from build123d import *

# Parameters (mm, degrees)
SCHIZZO1_R                   = 1.75
SCHIZZO1_R_2                 = 12.1
ESTRUSIONE_ESTRUSIONE1_DEPTH = 1
ESTRUSIONE_ESTRUSIONE2_START = -1.8
SCHIZZO2_R                   = 12.1
SCHIZZO2_R_2                 = 9
ESTRUSIONE_ESTRUSIONE2_DEPTH = 1.8


with BuildPart() as part:
    # Schizzo1 → Estrusione-Estrusione1 (new body)
    with BuildSketch(Plane.XY):
        with BuildLine():
            Line((-10.957517396, -18.677002221), (10.886206072, -18.677002221))
            ThreePointArc((10.886206072, -18.677002221), (14.572915114, -17.149917336), (16.1, -13.463208293))
            Line((16.1, -13.463208293), (16.1, 4.907883736))
            ThreePointArc((16.1, 4.907883736), (13.651991863, 12.73622021), (6.171311325, 16.1))
            Line((6.171311325, 16.1), (-6.171311325, 16.1))
            ThreePointArc((-6.171311325, 16.1), (-13.242379137, 13.171067812), (-16.171311325, 6.1))
            Line((-16.171311325, 6.1), (-16.171311325, -13.463208293))
            ThreePointArc((-16.171311325, -13.463208293), (-14.644226439, -17.149917336), (-10.957517396, -18.677002221))
        make_face()
        with Locations((0, -15.38859776)):
            Circle(SCHIZZO1_R, mode=Mode.SUBTRACT)
        with Locations((10.944459062, 10.817992606)):
            Circle(SCHIZZO1_R, mode=Mode.SUBTRACT)
        with Locations((-10.910719744, 10.851964601)):
            Circle(SCHIZZO1_R, mode=Mode.SUBTRACT)
        Circle(SCHIZZO1_R_2, mode=Mode.SUBTRACT)
    extrude(amount=ESTRUSIONE_ESTRUSIONE1_DEPTH)

    # Schizzo2 → Estrusione-Estrusione2 (add)
    with BuildSketch(Plane.XY.offset(1).offset(ESTRUSIONE_ESTRUSIONE2_START)):
        Circle(SCHIZZO2_R)
        Circle(SCHIZZO2_R_2, mode=Mode.SUBTRACT)
    extrude(amount=ESTRUSIONE_ESTRUSIONE2_DEPTH)


solid = part.part
Work out the finished part from the listing and answer in its coordinate system (mm). A direction names the side the tool comes from. Give positions to 0.01 mm unless a question says otherwise; leave off trailing zeros. Order: outer loops, then holes, each group sorted by start corner. A loop starts at its lowest first (then second) coordinate and runs counter-clockwise, first axis right, second up. Notation, with made-up numbers: (80.25, 27) -> (99.25, 27) arc R24 ccw to (99.25, 50) -> close; hole circle Ø4 at (-17.75, -39). An arc over 180 degrees is marked (long way). Answer as a JSON object with one key per item and string values. Group by question number.
1. Section D-D on x = -8 is taken. Determine the outline of the cut face in (y, z).
2. Section C-C on z = 0.35 is taken. Determine the outline of the cut face in (x, y).
3. A tool of negligible diameter and unlimited length cuts with its end or side. For faces 1 (the flat face through (0.1, 16.1, 0.5)), 2 (the flat face through (0, -13, 0)), 3 (the flat face through (16.1, -4.4, 0.5)), from which of +Z, -Z, +X, -X, +Y, -Y can it reach the whole face along a straight path? Write none if from no direction.
4. Consider line 1 along Y through (x, z) = (0, 0.5); line 2 along Z through (x, y) = (-9, -16); line 3 along X through (y, z) = (11, 0.65). Determine where each line is inside the solid, lowest interval first. Write a range as [from, to].
5. Section A-A on x = 0 is taken. Determine the outline of the cut face in (y, z).
6. Section B-B on y = 0 is taken. Determine the outline of the cut face in (x, z), plus the area to 3 significant figures.
7. Flat-ended cylindrical pins translate along their axes: pin 1 Ø3 at (x, y) = (-10.91, 10.85) entering from -Z; pin 2 Ø4 at (x, y) = (0, -15.39) entering from -Z; pin 3 Ø0.8 at (y, z) = (-8, 0.5) entering from +X. Find the tip coordinate at first contact, or state that the pin passes through.
8. The mould has two halves that part along X. Classify faces 4 (the cylindrical face through (-14.685, -17.109, 0.493)), 5 (the cylindrical face through (-0.228, -13.653, 0.493)), 6 (the flat face through (3, -9, 1)): released by +X, released by -X, zero draft, split by the parting line, or undercut.
Result sheet:
{
 "1": {"outline": "(-18.68, 0) -> (-9.08, 0) -> (-9.08, -0.8) -> (-4.12, -0.8) -> (-4.12, 1) -> (-18.68, 1) -> close; (4.12, -0.8) -> (9.08, -0.8) -> (9.08, 0) -> (15.93, 0) -> (15.93, 1) -> (4.12, 1) -> close"},
 "2": {"outline": "(-16.17, -13.46) arc R5.21 ccw to (-10.96, -18.68) -> (10.89, -18.68) arc R5.21 ccw to (16.1, -13.46) -> (16.1, 4.91) arc R10 ccw to (6.17, 16.1) -> (-6.17, 16.1) arc R10 ccw to (-16.17, 6.1) -> close; hole circle Ø3.5 at (-10.91, 10.85); hole circle Ø18 at (0, 0); hole circle Ø3.5 at (0, -15.39); hole circle Ø3.5 at (10.94, 10.82)"},
 "3": {"face 1": "+Z, -Z, +X, -X, +Y", "face 2": "-Z", "face 3": "+Z, -Z, +X, -Y"},
 "4": {"line 1": "y = [-18.68, -17.14], [-13.64, -9], [9, 16.1]", "line 2": "z = [0, 1]", "line 3": "x = [-14.89, -12.65], [-9.17, 9.2], [12.68, 14.89]"},
 "5": {"outline": "(-18.68, 0) -> (-17.14, 0) -> (-17.14, 1) -> (-18.68, 1) -> close; (-13.64, 0) -> (-12.1, 0) -> (-12.1, -0.8) -> (-9, -0.8) -> (-9, 1) -> (-13.64, 1) -> close; (9, -0.8) -> (12.1, -0.8) -> (12.1, 0) -> (16.1, 0) -> (16.1, 1) -> (9, 1) -> close"},
 "6": {"outline": "(-16.17, 0) -> (-12.1, 0) -> (-12.1, -0.8) -> (-9, -0.8) -> (-9, 1) -> (-16.17, 1) -> close; (9, -0.8) -> (12.1, -0.8) -> (12.1, 0) -> (16.1, 0) -> (16.1, 1) -> (9, 1) -> close", "area": "19.2 mm^2"},
 "7": {"pin 1": "passes through", "pin 2": "stops at z = 0", "pin 3": "stops at x = 16.1"},
 "8": {"face 4": "released by -X", "face 5": "undercut", "face 6": "zero draft"}
}
